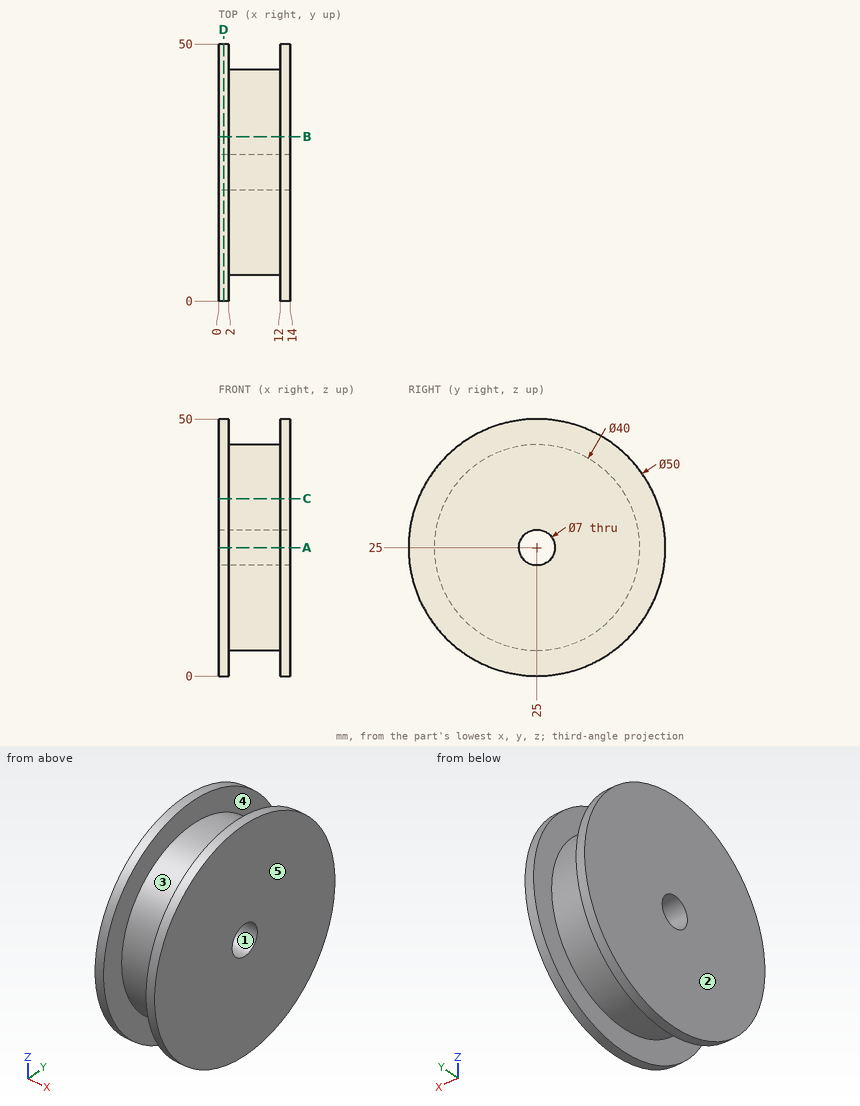
Part print with two shaded views. Sizes in mm from the minimum x, y, z corner. A direction names the side the tool comes from. Round coordinates to 2 decimals unless told otherwise and drop trailing zeros. Write each loop counter-clockwise with the first axis right and the second up, starting at its lowest first coordinate (ties: lowest second). Pieces come first, ordered by that corner, then holes. Notation, with made-up numbers: (41.25, 55.5) - (57.25, 55.5) arc R16 cw to (57.25, 85.5) - close; hole circle Ø10 at (86, 36.25). An arc over 180 degrees is marked (long way). Use CSV: the item, a comma, the result in double quotes.
Item 1: Flat gauge pins, fed straight in: P1, Ø2, axis at x = 5.5, z = 10.5, coming from the +Y side; P2, Ø11, axis at y = 25, z = 25, coming from the -X side; P3, Ø3, axis at x = 8.5, y = 22.5, coming from the -Z side (3 decimals); P4, Ø3, axis at x = 8.5, y = 16, coming from the +Z side. Where does each tip first touch, or does it go through?
Results list:
P1,"stops at y = 39.76"
P2,"stops at x = 0"
P3,"stops at z = 5.025"
P4,"stops at z = 43.54"
Item 2: Pull direction Y, two halves, no side cores. Call the marked faces 1, 2 and 3: pulls with the +Y half, pulls with the -Y half, needs draft (parallel to the pull), parting line crosses it, or undercut.
Results list:
face 1,"undercut"
face 2,"needs draft"
face 3,"parting line crosses it"
Item 3: Slice it at D-D, the plane x = 1. Write the cut outline in (y, z).
Results list:
outline,"circle Ø50 at (25, 25); hole circle Ø7 at (25, 25)"
Item 4: Wall check: L1, parallel to X at y = 28, z = 3; L2, parallel to Y at x = 7, z = 25; L3, parallel to Y at x = 10, z = 17.5. Give the ranges that are in metal, low to high.
Results list:
L1,"x = 0 to 2, 12 to 14"
L2,"y = 5 to 21.5, 28.5 to 45"
L3,"y = 6.46 to 43.54"
Item 5: Slice it at C-C, the plane z = 34.5. Write the cut outline in (x, y).
Results list:
outline,"(0, 1.88) - (2, 1.88) - (2, 7.4) - (12, 7.4) - (12, 1.88) - (14, 1.88) - (14, 48.12) - (12, 48.12) - (12, 42.6) - (2, 42.6) - (2, 48.12) - (0, 48.12) - close"
Item 6: Slice it at B-B, the plane y = 32. Write the cut outline in (x, z) (3 decimals), then the cut area to 3 significant figures.
Results list:
outline,"(0, 1) - (2, 1) - (2, 6.265) - (12, 6.265) - (12, 1) - (14, 1) - (14, 49) - (12, 49) - (12, 43.735) - (2, 43.735) - (2, 49) - (0, 49) - close"
area,"567 mm²"
Item 7: Slice it at A-A, the plane z = 25. Write the cut outline in (x, y).
Results list:
outline,"(0, 0) - (2, 0) - (2, 5) - (12, 5) - (12, 0) - (14, 0) - (14, 21.5) - (0, 21.5) - close; (0, 28.5) - (14, 28.5) - (14, 50) - (12, 50) - (12, 45) - (2, 45) - (2, 50) - (0, 50) - close"
Item 8: Tool access for the marked faces 4 and 5: list every direction of +Z, -Z, +X, -X, +Y, -Y with a clear straight run to the whole face (end or side of a thin tool).
Results list:
face 4,"none"
face 5,"+Z, -Z, +X, +Y, -Y"
